Solid Edge part; units mm, degrees
sketch "Sketch1" plane through (0, 0, 0) normal (0, -1, 0) x (1, 0, 0)
  circle A0 centre (0, 0) radius 21.5
extrude "Protrusion1" add sketch "Sketch1" against normal blind 5
sketch "Sketch2" plane through (0, 0, 0) normal (0, -1, 0) x (1, 0, 0)
  circle A0 centre (0, 0) radius 21.5
  circle A1 centre (0, 0) radius 18.75
extrude "ExtrudedProtrusion_2" add sketch "Sketch2" along normal blind 21.4
sketch "Sketch3" plane through (0, -21.4, 0) normal (0, -1, 0) x (1, 0, 0)
  line L0 (-31.1127, 22.6274) -> (-18.8414, 10.3562)
  arc A0 (-18.8414, 10.3562) -> (-10.3562, 18.8414) centre (0, 0) cw
  line L1 (-22.6274, 31.1127) -> (-10.3562, 18.8414)
  line L2 (-22.6274, 31.1127) -> (-31.1127, 22.6274)
  line L3 (-31.1127, -22.6274) -> (-18.8414, -10.3562)
  arc A1 (-10.3562, -18.8414) -> (-18.8414, -10.3562) centre (0, 0) cw
  line L4 (-22.6274, -31.1127) -> (-10.3562, -18.8414)
  line L5 (-31.1127, -22.6274) -> (-22.6274, -31.1127)
  line L6 (22.6274, -31.1127) -> (10.3562, -18.8414)
  arc A2 (18.8414, -10.3562) -> (10.3562, -18.8414) centre (0, 0) cw
  line L7 (31.1127, -22.6274) -> (18.8414, -10.3562)
  line L8 (31.1127, -22.6274) -> (22.6274, -31.1127)
  line L9 (31.1127, 22.6274) -> (18.8414, 10.3562)
  line L10 (22.6274, 31.1127) -> (10.3562, 18.8414)
  line L11 (31.1127, 22.6274) -> (22.6274, 31.1127)
  arc A3 (10.3562, 18.8414) -> (18.8414, 10.3562) centre (0, 0) cw
extrude "ExtrudedProtrusion_3" add sketch "Sketch3" against normal blind 6
sketch "Sketch4" plane through (0, -21.4, 0) normal (0, -1, 0) x (0.7071, 0, -0.7071)
  circle A0 centre (-31.7502, 0) radius 3.15
  circle A1 centre (0, 31.75) radius 3.15
  circle A2 centre (31.75, 0) radius 3.15
  circle A3 centre (0, -31.75) radius 3.15
extrude "Cutout1" cut sketch "Sketch4" against normal up to next
sketch "Sketch5" plane through (0, 5, 0) normal (0, 1, 0) x (-1, 0, 0)
  circle A0 centre (7.75, 13.43) radius 1.6
  circle A1 centre (-7.75, 13.43) radius 1.6
  circle A2 centre (-15.5, 0) radius 1.6
  circle A3 centre (15.5, 0) radius 1.6
  circle A4 centre (7.75, -13.43) radius 1.6
  circle A5 centre (-7.75, -13.43) radius 1.6
  circle A6 centre (0, -7) radius 6.1
extrude "Cutout2" cut sketch "Sketch5" against normal up to next
chamfer "Chamfer_1" distance 1.87 angle 45 6 edges at (17.1, 5, 0) (9.35, 5, 13.43) (-6.15, 5, 13.43) (-13.9, 5, 0) (-6.15, 5, -13.43) (9.35, 5, -13.43)
chamfer "Chamfer_2" distance 5 angle 45 4 edges at (-15.2028, -15.4, -15.2028) (15.2028, -15.4, -15.2028) (15.2028, -15.4, 15.2028) (-15.2028, -15.4, 15.2028)
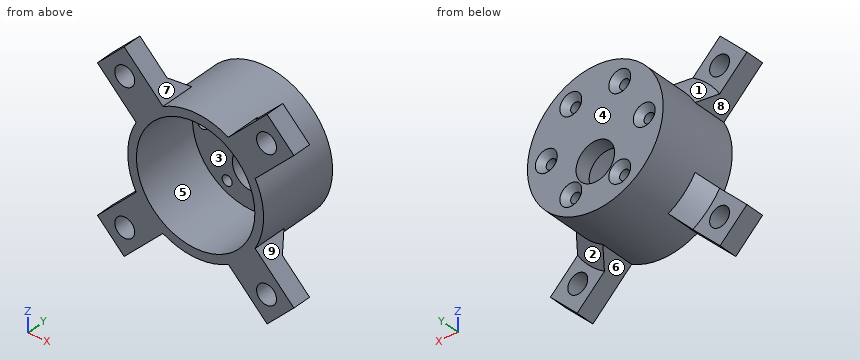
Work out the finished part from the listing and answer in its coordinate system (mm). Face numbers are marked on the shaded views. A direction names the side the tool comes from. Give positions to 0.01 mm unless a question says otherwise; leave off trailing zeros. Loops run counter-clockwise (first coordinate to the right, second up) from the corner with the lowest first, then second, coordinate; pieces in that order, holes last. Notation, with made-up numbers: M -11.75,73 L 25.25,73 A16 cw 25.25,99 Z; hole C 52.5,10.5 d5. An arc over 180 degrees is marked long. Use CSV: the item, a comma, the result in double quotes.
1) Determine the mould class of the marked faces 1, 2, 3 and 4 for opening direction Z: released by +Z, released by -Z, zero draft, split by the parting line, or undercut.
Answer:
face 1,"released by +Z"
face 2,"released by -Z"
face 3,"undercut"
face 4,"zero draft"
2) Consider L1, parallel to Z at x = 0, y = -12.75; L2, parallel to Z at x = 0, y = 1.25; L3, parallel to Z at x = 7.75, y = 0.7. Determine where each line is inside the solid, lowest interval first.
Answer:
L1,"-21.5 to -18.75, 18.75 to 21.5"
L2,"-21.5 to -13.1, -0.9 to 21.5"
L3,"-20.05 to -15.03, -11.83 to 11.83, 15.03 to 20.05"
3) Which of the six approach directions +Z, -Z, +X, -X, +Y, -Y give full straight-line access (tool end or side, diameter ignored) to the marked faces 5, 6, 7, 8 and 9?
Answer:
face 5,"-Y"
face 6,"-Z, +Y, -Y"
face 7,"+Z, +Y, -Y"
face 8,"-X, +Y, -Y"
face 9,"+X, +Y, -Y"
4) Find section D-D on y = -14.25. Write down the section's boundary in (x, z), plus the area to 3 significant figures.
Answer:
outline,"M -21.66,-13.17 A25.35 ccw -13.17,-21.66 L -10.36,-18.84 A21.5 ccw 10.36,-18.84 L 13.17,-21.66 A25.35 ccw 21.66,-13.17 L 18.84,-10.36 A21.5 ccw 18.84,10.36 L 21.66,13.17 A25.35 ccw 13.17,21.66 L 10.36,18.84 A21.5 ccw -10.36,18.84 L -13.17,21.66 A25.35 ccw -21.66,13.17 L -18.84,10.36 A21.5 ccw -18.84,-10.36 Z; hole C 0,0 d37.5"
area,"535 mm^2"
5) Find section B-B on x = 7.75. Write down the section's boundary in (y, z).
Answer:
outline,"M -21.4,-20.05 L 5,-20.05 L 5,-16.9 L 3.13,-15.03 L 0,-15.03 L 0,-17.07 L -21.4,-17.07 Z; M -21.4,17.07 L 0,17.07 L 0,15.03 L 3.13,15.03 L 5,16.9 L 5,20.05 L -21.4,20.05 Z; M 0,-11.83 L 3.13,-11.83 L 5,-9.96 L 5,9.96 L 3.13,11.83 L 0,11.83 Z"
6) Find section C-C on z = -7. Write down the section's boundary in (x, y).
Answer:
outline,"M -20.33,-21.4 L -17.39,-21.4 L -17.39,0 L -6.1,0 L -6.1,5 L -20.33,5 Z; M 6.1,0 L 17.39,0 L 17.39,-21.4 L 20.33,-21.4 L 20.33,5 L 6.1,5 Z"
7) Find section A-A on x = 0. Write down the section's boundary in (y, z).
Answer:
outline,"M -21.4,-21.5 L 5,-21.5 L 5,-13.1 L 0,-13.1 L 0,-18.75 L -21.4,-18.75 Z; M -21.4,18.75 L 0,18.75 L 0,-0.9 L 5,-0.9 L 5,21.5 L -21.4,21.5 Z"
8) Given P1, Ø8, axis at x = -22.45, z = 22.45, coming from the -Y side; P2, Ø3, axis at x = -15.5, z = 0, coming from the -Y side; P3, Ø6, axis at x = 2, y = -11.5, coming from the +Z side; P4, Ø1.5, axis at y = -15.5, z = 3.5, coming from the +X side, each flat-ended and moving along its own axis, determine where each tip first touches the part or whether it passes through.
Answer:
P1,"y = -21.4"
P2,"through"
P3,"z = 21.5"
P4,"x = 21.32"
